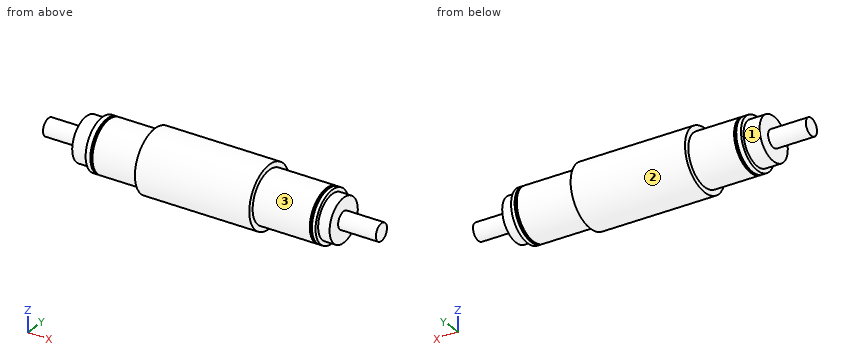
from build123d import *

# Parameters (mm, degrees)
SCHIZZO2_W   = 1.6
SCHIZZO2_H   = 6.8
SCHIZZO2_W_2 = 1.85
SCHIZZO2_H_2 = 1.25


with BuildPart() as part:
    # Schizzo1 → Rivoluzione1 (revolve)
    with BuildSketch(Plane.XY, mode=Mode.PRIVATE) as rivoluzione1_sk:
        Polygon((0, 0), (291, 0), (291, 7.5), (258, 7.5), (258, 19), (248, 19), (248, 22.5), (193, 22.5), (193, 27), (93, 27), (93, 22.5), (47, 22.5), (47, 19), (33, 19), (33, 7.5), (0, 7.5), align=None)
    revolve(rivoluzione1_sk.sketch.rotate(Axis((0, 0, 0), (1, 0, 0)), 90), axis=Axis((0, 0, 0), (1, 0, 0)))

    # Schizzo2 → Taglia-Rivoluzione1 (revolve, cut)
    with BuildSketch(Plane.XY, mode=Mode.PRIVATE) as taglia_rivoluzione1_sk:
        with Locations((5.2, 10.9)):
            Rectangle(SCHIZZO2_W, SCHIZZO2_H)
        with Locations((52.075, 21.875)):
            Rectangle(SCHIZZO2_W_2, SCHIZZO2_H_2)
        with Locations((243.925, 21.875)):
            Rectangle(SCHIZZO2_W_2, SCHIZZO2_H_2)
        with Locations((285.8, 10.9)):
            Rectangle(SCHIZZO2_W, SCHIZZO2_H)
    revolve(taglia_rivoluzione1_sk.sketch.rotate(Axis((0, 0, 0), (1, 0, 0)), 90), axis=Axis((0, 0, 0), (1, 0, 0)), mode=Mode.SUBTRACT)


solid = part.part
CAD build for the part. Positions are in the model's coordinates, mm. Face numbers are marked on the shaded views. A direction names the side the tool comes from. Round coordinates to 2 decimals unless told otherwise and drop trailing zeros. Loops run counter-clockwise (first coordinate to the right, second up) from the corner with the lowest first, then second, coordinate; pieces in that order, holes last. Notation, with made-up numbers: (79.25, 24) - (114.25, 24) arc R29 ccw to (114.25, 52) - close; hole circle Ø5 at (47, -15). An arc over 180 degrees is marked (long way). Put each result on its own line as item: value.
1. Pin check, flat tips, straight feed: P1, Ø4, axis at y = -20.5, z = -3.5, coming from the -X side; P2, Ø13.5, axis at y = -5, z = 8.5, coming from the -X side; P3, Ø2, axis at x = 256, y = 4.5, coming from the +Z side; P4, Ø1.5, axis at x = 252, y = -21.5, coming from the -Z side. Stop position of each tip, or through.
Geometry check:
P1: x = 33
P2: x = 0
P3: z = 18.67
P4: through
2. Slice it at B-B on x = 173. List the corners of the cut face in (y, z).
Geometry check:
outline: circle Ø54 at (0, 0)
3. Slice it at A-A on x = 38. List the corners of the cut face in (y, z).
Geometry check:
outline: circle Ø38 at (0, 0)
4. 3-axis set-ups, long thin cutter, end or side, ignore diameter. For the marked faces 1, 2 and 3: which of +Z, -Z, +X, -X, +Y, -Y reach the whole face in a straight line?
Geometry check:
face 1: -X
face 2: +X, -X
face 3: +X
5. Wall check: line 1 (X direction, y = -2.5, z = -7.5); line 2 (Z direction, x = 118, y = 1.5); line 3 (X direction, y = 10.5, z = -23). Give the ranges that are in metal, low to high.
Geometry check:
line 1: 33 to 258
line 2: -26.96 to 26.96
line 3: 93 to 193
